```python
from build123d import *

# Parameters (mm, degrees)
SKETCH1_W           = 20
SKETCH1_H           = 23
BOSS_EXTRUDE1_DEPTH = 34
SKETCH2_R           = 0.8
CUT_EXTRUDE1_DEPTH  = 24
SKETCH3_R           = 8
SKETCH3_R_2         = 0.8
BOSS_EXTRUDE2_DEPTH = 3
SKETCH4_W           = 4
SKETCH4_H           = 11
CUT_EXTRUDE2_DEPTH  = 9


with BuildPart() as part:
    # Sketch1 → Boss-Extrude1 (new body)
    with BuildSketch(Plane(origin=(0, 0, 0), x_dir=(1, 0, 0), z_dir=(0, 1, 0))):
        with Locations((10, 11.5)):
            Rectangle(SKETCH1_W, SKETCH1_H)
    extrude(amount=BOSS_EXTRUDE1_DEPTH)

    # Sketch2 → Cut-Extrude1 (cut, through all)
    with BuildSketch(Plane.XY):
        with Locations((2, 32)):
            Circle(SKETCH2_R)
        with Locations((18, 32)):
            Circle(SKETCH2_R)
        with Locations((18, 2)):
            Circle(SKETCH2_R)
        with Locations((2, 2)):
            Circle(SKETCH2_R)
    extrude(amount=-CUT_EXTRUDE1_DEPTH, mode=Mode.SUBTRACT)

    # Sketch3 → Boss-Extrude2 (add)
    with BuildSketch(Plane.XY):
        with Locations((10, 9.5)):
            Circle(SKETCH3_R)
        with Locations((10, 15.5)):
            Circle(SKETCH3_R_2, mode=Mode.SUBTRACT)
        with Locations((4, 9.5)):
            Circle(SKETCH3_R_2, mode=Mode.SUBTRACT)
        with Locations((10, 3.5)):
            Circle(SKETCH3_R_2, mode=Mode.SUBTRACT)
        with Locations((16, 9.5)):
            Circle(SKETCH3_R_2, mode=Mode.SUBTRACT)
    extrude(amount=BOSS_EXTRUDE2_DEPTH)

    # Sketch4 → Cut-Extrude2 (cut)
    with BuildSketch(Plane(origin=(0, 0, -23), x_dir=(-1, 0, 0), z_dir=(0, 0, -1))):
        with Locations((-18, 18.5)):
            Rectangle(SKETCH4_W, SKETCH4_H)
        with Locations((-2, 18.5)):
            Rectangle(SKETCH4_W, SKETCH4_H)
    extrude(amount=-CUT_EXTRUDE2_DEPTH, mode=Mode.SUBTRACT)


solid = part.part
```
Geometry check sheet. Reference: the model listing, model coordinates, mm. A direction names the side the tool comes from. Round coordinates to 2 decimals unless told otherwise and drop trailing zeros. Loops run counter-clockwise (first coordinate to the right, second up) from the corner with the lowest first, then second, coordinate; pieces in that order, holes last. Notation, with made-up numbers: M -20.75,4 L 9.25,4 A21 cw 9.25,39 Z; hole C 8.25,89.25 d9. An arc over 180 degrees is marked long. Return JSON: item names as keys, results as strings. Group by question number.
(1) Set-up check for faces 1 (the face through (10, 0, -12)), 2 (the face through (18, 24, -19)), 3 (the face through (0, 17, -11)), 4 (the face through (15.896, 10.293, 1.479)), 5 (the face through (2, 24, -19)): record each of +Z, -Z, +X, -X, +Y, -Y from which the full face is reachable in a straight line by a thin tool's end or side.
(2) Section check C-C, the plane x = 5.5. Enter the section's corners in (y, z).
(3) Section check D-D, the plane y = 21. Enter the section's corners in (x, z).
(4) Scan lines: line 1 along Y through (x, z) = (18, -13.5); line 2 along X through (y, z) = (32, -5); line 3 along Y through (x, z) = (10, 1.6). Record each from-to range of solid material in increasing order. Write a range as [from, to].
(5) Section check A-A, the plane z = -18. Enter the section's corners in (x, y).
(6) Go/stop test with flat-tipped pins: pin 1 (2 mm diameter, centred on y = 15.5, z = -16.5, fed in from -X); pin 2 (4.5 mm diameter, centred on y = 19, z = -17, fed in from +X); pin 3 (1 mm diameter, centred on x = 10, y = 3.5, fed in from +Z). Record where each tip stops, or that it passes through.
(7) Mould release check, pull along X, two halves, no side actions. Record for faces 6 (the face through (17.2, 2, -11.3)), 7 (the face through (10, 3, 0)), 8 (the face through (10, 21, 0)), 9 (the face through (4, 18, -19)): pulls with the +X half, pulls with the -X half, needs draft (parallel to the pull), parting line crosses it, or undercut.
(8) Section check B-B, the plane y = 32. Enter the section's corners in (x, z), and give its area (3 significant figures).
Data:
{
 "1": {"face 1": "+Z, -Z, +X, -X, -Y", "face 2": "-Z, +X", "face 3": "+Z, -Z, -X, +Y, -Y", "face 4": "+Z", "face 5": "-Z, -X"},
 "2": {"outline": "M 0,-23 L 34,-23 L 34,0 L 16.11,0 L 16.11,3 L 2.89,3 L 2.89,0 L 0,0 Z"},
 "3": {"outline": "M 0,-14 L 4,-14 L 4,-23 L 16,-23 L 16,-14 L 20,-14 L 20,0 L 0,0 Z"},
 "4": {"line 1": "[0, 1.2], [2.8, 31.2], [32.8, 34]", "line 2": "[0, 1.2], [2.8, 17.2], [18.8, 20]", "line 3": "[1.5, 2.7], [4.3, 14.7], [16.3, 17.5]"},
 "5": {"outline": "M 0,0 L 20,0 L 20,13 L 16,13 L 16,24 L 20,24 L 20,34 L 0,34 L 0,24 L 4,24 L 4,13 L 0,13 Z; hole C 2,2 d1.6; hole C 2,32 d1.6; hole C 18,2 d1.6; hole C 18,32 d1.6"},
 "6": {"pin 1": "x = 4", "pin 2": "x = 16", "pin 3": "z = 0"},
 "7": {"face 6": "undercut", "face 7": "undercut", "face 8": "needs draft", "face 9": "pulls with the -X half"},
 "8": {"outline": "M 0,-23 L 1.2,-23 L 1.2,0 L 0,0 Z; M 2.8,-23 L 17.2,-23 L 17.2,0 L 2.8,0 Z; M 18.8,-23 L 20,-23 L 20,0 L 18.8,0 Z", "area": "386 mm²"}
}
